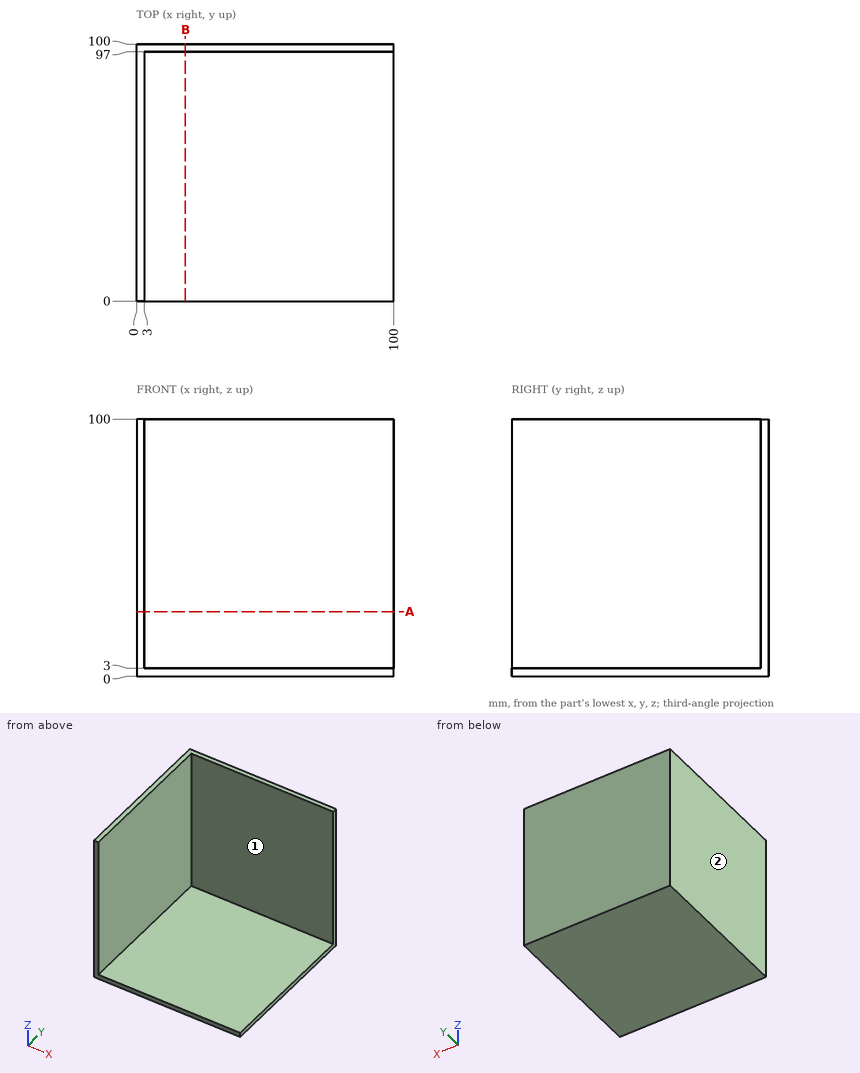
The figure shows three views and two pictorial views of one solid part (mm, origin at its lowest corner). Answer the questions. A direction names the side the tool comes from. Give positions to 0.01 mm unless a question says otherwise; leave off trailing zeros. Write each loop counter-clockwise with the first axis right and the second up, starting at its lowest first coordinate (ties: lowest second). Pieces come first, ordered by that corner, then holes. Notation, with made-up numbers: (-31.75, 64.5) - (-19.75, 64.5) arc R14 cw to (-19.75, 71.5) - close; hole circle Ø5 at (-17.75, -9.75). An arc over 180 degrees is marked (long way). Use one line per item in the form item = value.
1. For the marked faces 1 and 2, determine the directions among +Z, -Z, +X, -X, +Y, -Y from which every point of the face is accessible in a straight line to the end or side of a thin tool.
Filled in:
face_1 = +Z, +X, -Y
face_2 = +Z, -Z, -X, +Y, -Y
2. Consider L1, parallel to Y at x = 73.5, z = 74; L2, parallel to Z at x = 58.5, y = 18.5. Determine where each line is inside the solid, lowest interval first.
Filled in:
L1 = 97 to 100
L2 = 0 to 3
3. A cutting plane is placed at A-A (z = 25). Write down the section's boundary in (x, y).
Filled in:
outline = (0, 0) - (3, 0) - (3, 97) - (100, 97) - (100, 100) - (0, 100) - close
4. A cutting plane is placed at B-B (x = 19). Write down the section's boundary in (y, z).
Filled in:
outline = (0, 0) - (100, 0) - (100, 100) - (97, 100) - (97, 3) - (0, 3) - close
5. Each of these flat-tipped pins is pushed along its axis until it touches: pin 1 Ø6 at (y, z) = (20, 23) entering from +X; pin 2 Ø2 at (x, z) = (74, 32.5) entering from -Y; pin 3 Ø5 at (x, y) = (66, 65.5) entering from +Z. Where does it stop, or does it pass through?
Filled in:
pin_1 = 3
pin_2 = 97
pin_3 = 3
